The listing builds one solid part. Answer for the finished solid, in the listing's coordinates (mm). A direction names the side the tool comes from. Coordinates: 2 decimals unless noted, no trailing zeros. Order: outer loops, then holes, each group sorted by start corner. A loop starts at its lowest first (then second) coordinate and runs counter-clockwise, first axis right, second up.
from build123d import *

# Parameters (mm, degrees)
SCHIZZO1_W                   = 56
SCHIZZO1_H                   = 56
ESTRUSIONE_ESTRUSIONE1_DEPTH = 41
SCHIZZO2_R                   = 2.5
TAGLIO_ESTRUSIONE1_DEPTH     = 41
SCHIZZO3_R                   = 15
ESTRUSIONE_ESTRUSIONE3_DEPTH = 2
SCHIZZO4_R                   = 2.5
ESTRUSIONE_ESTRUSIONE4_DEPTH = 19.3
SCHIZZO5_R                   = 10.5
TAGLIO_ESTRUSIONE2_DEPTH     = 36
CONG_1_R                     = 5


with BuildPart() as part:
    # Schizzo1 → Estrusione-Estrusione1 (new body)
    with BuildSketch(Plane(origin=(0, 0, 0), x_dir=(1, 0, 0), z_dir=(0, 1, 0))):
        Rectangle(SCHIZZO1_W, SCHIZZO1_H)
    extrude(amount=ESTRUSIONE_ESTRUSIONE1_DEPTH)

    # Schizzo2 → Taglio-Estrusione1 (cut)
    with BuildSketch(Plane(origin=(0, 41, 0), x_dir=(1, 0, 0), z_dir=(0, 1, 0))):
        with Locations(Location((-23.5, 23.5, 0), (0, 0, 270))):
            Circle(SCHIZZO2_R)
        with Locations(Location((23.5, 23.5, 0), (0, 0, 270))):
            Circle(SCHIZZO2_R)
        with Locations(Location((23.5, -23.5, 0), (0, 0, 270))):
            Circle(SCHIZZO2_R)
        with Locations(Location((-23.5, -23.5, 0), (0, 0, 270))):
            Circle(SCHIZZO2_R)
    extrude(amount=-TAGLIO_ESTRUSIONE1_DEPTH, mode=Mode.SUBTRACT)

    # Schizzo3 → Estrusione-Estrusione3 (add)
    with BuildSketch(Plane(origin=(0, 41, 0), x_dir=(1, 0, 0), z_dir=(0, 1, 0))):
        with Locations(Location((0, 0, 0), (0, 0, 90))):
            Circle(SCHIZZO3_R)
    extrude(amount=ESTRUSIONE_ESTRUSIONE3_DEPTH)

    # Schizzo4 → Estrusione-Estrusione4 (add)
    with BuildSketch(Plane(origin=(0, 43, 0), x_dir=(1, 0, 0), z_dir=(0, 1, 0))):
        with Locations(Location((0, 0, 0), (0, 0, 270))):
            Circle(SCHIZZO4_R)
    extrude(amount=ESTRUSIONE_ESTRUSIONE4_DEPTH)

    # Schizzo5 → Taglio-Estrusione2 (cut)
    with BuildSketch(Plane.XZ):
        with Locations((-28, 28)):
            Circle(SCHIZZO5_R)
        with Locations((28, 28)):
            Circle(SCHIZZO5_R)
        with Locations((28, -28)):
            Circle(SCHIZZO5_R)
        with Locations((-28, -28)):
            Circle(SCHIZZO5_R)
    extrude(amount=-TAGLIO_ESTRUSIONE2_DEPTH, mode=Mode.SUBTRACT)

    # Congé1
    # the kernel refuses this fillet: 5 mm, written as the material it takes off along each edge
    with BuildSketch(Plane(origin=(40.5, 41, -28), x_dir=(0, 0, 1), z_dir=(-1, 0, 0)), Plane(origin=(-28, 41, -40.5), x_dir=(1, 0, 0), z_dir=(0, 0, 1))) as cong_1_piece_1:
        with BuildLine():
            CenterArc((CONG_1_R, -CONG_1_R), CONG_1_R, 90, 90)
            Line((0, -CONG_1_R), (0, 0))
            Line((0, 0), (CONG_1_R, 0))
        make_face()
    extrude(amount=81, mode=Mode.SUBTRACT)
    with BuildSketch(Plane(origin=(-40.5, 41, 28), x_dir=(0, -1, 0), z_dir=(1, 0, 0)), Plane(origin=(28, 41, 40.5), x_dir=(0, -1, 0), z_dir=(0, 0, -1))) as cong_1_piece_2:
        with BuildLine():
            CenterArc((CONG_1_R, CONG_1_R), CONG_1_R, 180, 90)
            Line((0, CONG_1_R), (0, 0))
            Line((0, 0), (CONG_1_R, 0))
        make_face()
    extrude(amount=81, mode=Mode.SUBTRACT)


solid = part.part
(1) Find section C-C on z = 0. Determine the outline of the cut face in (x, y), then the cut area to 3 significant figures.
(2) Find the intervals of material crossed by probe 1 along Z at (x, y) = (-23.5, 39.1); probe 2 along Z at (x, y) = (-23.5, 37.7), in increasing order.
(3) Given pin 1 Ø3 at (x, z) = (-23.5, 23.5) entering from +Y; pin 2 Ø3 at (x, z) = (-23, 22) entering from -Y; pin 3 Ø12 at (x, z) = (5, 16.5) entering from +Y, each flat-ended and moving along its own axis, determine where each tip first touches the part or whether it passes through.
(4) Find section D-D on x = -16.5. Determine the outline of the cut face in (y, z).
(5) Find section B-B on x = 0. Determine the outline of the cut face in (y, z).
(6) The mould has two halves that part along X. Classify faces 5 (the flat face through (-26.3, 36, -23.8)), 6 (the cylindrical face through (-21.39, 38.53, -22.16)), 7 (the cylindrical face through (20.49, 17.75, 20.66)): pulls with the +X half, pulls with the -X half, needs draft (parallel to the pull), parting line crosses it, or undercut.
(7) A tool of negligible diameter and unlimited length cuts with its end or side. For faces 1 (the cylindrical face through (-0.66, 41.986, 14.985)), 2 (the flat face through (-24, 36, 26.3)), 3 (the cylindrical face through (-20.49, 17.75, -20.66)), 4 (the flat face through (23.8, 36, 26.3)), from which of +Z, -Z, +X, -X, +Y, -Y can it reach the whole face along a straight path? Write none if from no direction.
(8) Find section A-A on y = 24.5. Determine the outline of the cut face in (x, z).
Resolved:
1. outline: (-28, 0) - (28, 0) - (28, 36) arc R5 ccw to (23, 41) - (15, 41) - (15, 43) - (2.5, 43) - (2.5, 62.3) - (-2.5, 62.3) - (-2.5, 43) - (-15, 43) - (-15, 41) - (-23, 41) arc R5 ccw to (-28, 36) - close
1. area: 2,440 mm2
2. probe 1: z = -26.92 to -26, -21 to 21, 26 to 26.92
2. probe 2: z = -27.7 to -26, -21 to 21, 26 to 27.7
3. pin 1: passes through
3. pin 2: stops at y = 36
3. pin 3: stops at y = 43
4. outline: (0, -28) - (36, -28) arc R5 ccw to (41, -23) - (41, 23) arc R5 ccw to (36, 28) - (0, 28) - close
5. outline: (0, -28) - (36, -28) arc R5 ccw to (41, -23) - (41, -15) - (43, -15) - (43, -2.5) - (62.3, -2.5) - (62.3, 2.5) - (43, 2.5) - (43, 15) - (41, 15) - (41, 23) arc R5 ccw to (36, 28) - (0, 28) - close
6. face 5: needs draft
6. face 6: undercut
6. face 7: pulls with the +X half
7. face 1: +Y
7. face 2: +Z, -X, -Y
7. face 3: -Z, -X, -Y
7. face 4: +Z, +X, -Y
8. outline: (-28, -17.5) arc R10.5 cw to (-17.5, -28) - (17.5, -28) arc R10.5 cw to (28, -17.5) - (28, 17.5) arc R10.5 cw to (17.5, 28) - (-17.5, 28) arc R10.5 cw to (-28, 17.5) - close
